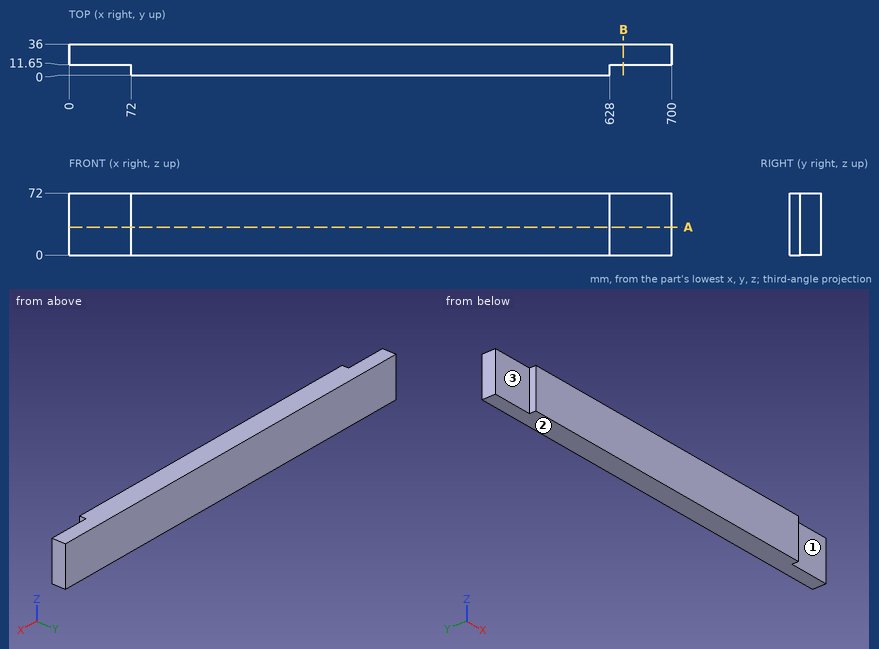
Input: dimensioned drawing with shaded views. Units: mm. Origin: part minimum x, y, z. A direction names the side the tool comes from. Round coordinates to 2 decimals unless told otherwise and drop trailing zeros. Order: outer loops, then holes, each group sorted by start corner. A loop starts at its lowest first (then second) coordinate and runs counter-clockwise, first axis right, second up.
Q1. Section B-B, the plane x = 643.5. Output: boundary loops of the cut face in (y, z), and give its area (3 significant figures).
Result sheet:
outline: (11.65, 0) - (36, 0) - (36, 72) - (11.65, 72) - close
area: 1,750 mm2
Q2. Material intervals for probe 1 along Y at (x, z) = (58, 21); probe 2 along X at (y, z) = (11.5, 22), sorted ascending.
Result sheet:
probe 1: y = 11.65 to 36
probe 2: x = 72 to 628
Q3. Pin query (flat end, axial travel): pin 1 (10 mm diameter, centred on x = 530, y = 15, fed in from -Z); pin 2 (6 mm diameter, centred on y = 6, z = 28.5, fed in from +X); pin 3 (13 mm diameter, centred on y = 4.5, z = 19, fed in from -X). Return the tip coordinate at first contact, or that it passes through.
Result sheet:
pin 1: stops at z = 0
pin 2: stops at x = 628
pin 3: stops at x = 72
Q4. Section A-A, the plane z = 32.5. Output: boundary loops of the cut face in (x, y).
Result sheet:
outline: (0, 11.65) - (72, 11.65) - (72, 0) - (628, 0) - (628, 11.65) - (700, 11.65) - (700, 36) - (0, 36) - close
Q5. Access query for the marked faces 1, 2 and 3. Directions: +Z, -Z, +X, -X, +Y, -Y. A direction counts if a zero-diameter tool reaches every point of the face in a straight line with its end or side. Return the directions, or none.
Result sheet:
face 1: +Z, -Z, +X, -Y
face 2: -Z, +X, -X, +Y, -Y
face 3: +Z, -Z, -X, -Y
